```python
from build123d import *

# Parameters (mm, degrees)
SKETCH_W               = 9
SKETCH_H               = 250
PAD_DEPTH              = 6.5
SKETCH001_R            = 1.75
POCKET_DEPTH           = 6.5
LINEARPATTERN_COUNT    = 13
LINEARPATTERN_PITCH    = 20
SKETCH002_R            = 3
POCKET001_DEPTH        = 3.5
LINEARPATTERN001_COUNT = 13
LINEARPATTERN001_PITCH = 20
SKETCH005_W            = 20
SKETCH005_H            = 28.9
SKETCH005_R            = 1.75
PAD002_DEPTH           = 8


with BuildPart() as part:
    # Sketch → Pad (new body)
    with BuildSketch(Plane.XY):
        with Locations((0, 125)):
            Rectangle(SKETCH_W, SKETCH_H)
    extrude(amount=-PAD_DEPTH)

    # Sketch001 → Pocket (cut)
    with BuildSketch(Plane.XY):
        with Locations((0, 5)):
            Circle(SKETCH001_R)
    pocket = extrude(amount=-POCKET_DEPTH, mode=Mode.SUBTRACT)

    # LinearPattern: Pocket ×13
    with Locations(*[(0, i * LINEARPATTERN_PITCH, 0) for i in range(1, LINEARPATTERN_COUNT)]):
        add(pocket, mode=Mode.SUBTRACT)

    # Sketch002 → Pocket001 (cut)
    with BuildSketch(Plane.XY):
        with Locations((0, 5)):
            Circle(SKETCH002_R)
    pocket001 = extrude(amount=-POCKET001_DEPTH, mode=Mode.SUBTRACT)

    # LinearPattern001: Pocket001 ×13
    with Locations(*[(0, i * LINEARPATTERN001_PITCH, 0) for i in range(1, LINEARPATTERN001_COUNT)]):
        add(pocket001, mode=Mode.SUBTRACT)

    # Sketch005 → Pad002 (join)
    with BuildSketch(Plane.XY.offset(-4.5)):
        with Locations((0, 132.225)):
            Rectangle(SKETCH005_W, SKETCH005_H)
        with Locations((-7.5, 137.225)):
            Circle(SKETCH005_R, mode=Mode.SUBTRACT)
        with Locations((7.5, 137.225)):
            Circle(SKETCH005_R, mode=Mode.SUBTRACT)
        with Locations((7.5, 127.225)):
            Circle(SKETCH005_R, mode=Mode.SUBTRACT)
        with Locations((-7.5, 127.225)):
            Circle(SKETCH005_R, mode=Mode.SUBTRACT)
    extrude(amount=PAD002_DEPTH)


solid = part.part
```
Part model, mm, in its own coordinate system. A direction names the side the tool comes from. Coordinates: 2 decimals unless noted, no trailing zeros. Order: outer loops, then holes, each group sorted by start corner. A loop starts at its lowest first (then second) coordinate and runs counter-clockwise, first axis right, second up. Notation, with made-up numbers: (0.5, 57.25) - (20.5, 57.25) arc R20 ccw to (20.5, 65.25) - close; hole circle Ø8 at (16, 68.25). An arc over 180 degrees is marked (long way). Return JSON: item names as keys, results as strings. Group by question number.
Item 1: Pin check, flat tips, straight feed: pin 1 (3 mm diameter, centred on x = -1.5, y = 164, fed in from +Z); pin 2 (4 mm diameter, centred on x = 7.5, y = 84, fed in from +Z); pin 3 (1.7 mm diameter, centred on x = 0, y = 145, fed in from -Z); pin 4 (5.5 mm diameter, centred on x = 0, y = 205, fed in from +Z). Stop position of each tip, or through.
Item 2: Cut at A-A (z = 1.75). List the corners of the cut face in (x, y) (3 decimals), plus the area to 3 significant figures.
Item 3: Drill centre lines: probe 1 along Y at (x, z) = (-7.5, 1.75) (3 decimals); probe 2 along X at (y, z) = (185, -5.05); probe 3 along X at (y, z) = (137.5, -3). Where is each one in solid material? Low to high. Write a range as from..to.
Item 4: Which spindle directions (+Z, -Z, +X, -X, +Y, -Y) get a long thin tool onto all of the face, cutting with end or side? Do faces 4 (the face through (2, 245, -3.5)), 5 (the face through (0, 127, -6.5)), 6 (the face through (0, 199, 0)). Say none if no direction does.
Item 5: Pull direction Y, two halves, no side cores. Call faces 1 (the face through (10, 132, -1)), 2 (the face through (0, 250, -3)), 3 (the face through (2, 5, -3.5)): pulls with the +Y half, pulls with the -Y half, needs draft (parallel to the pull), parting line crosses it, or undercut.
Item 6: Cut at B-B (y = 175). List the corners of the cut face in (x, z), plus the area to 3 significant figures.
Check values:
{
 "1": {"pin 1": "stops at z = 0", "pin 2": "passes through", "pin 3": "stops at z = -4.5", "pin 4": "stops at z = -3.5"},
 "2": {"outline": "(-10, 117.775) - (10, 117.775) - (10, 146.675) - (-10, 146.675) - close; hole circle Ø3.5 at (-7.5, 127.225); hole circle Ø3.5 at (-7.5, 137.225); hole circle Ø3.5 at (7.5, 127.225); hole circle Ø3.5 at (7.5, 137.225)", "area": "540 mm2"},
 "3": {"probe 1": "y = 117.775..125.475, 128.975..135.475, 138.975..146.675", "probe 2": "x = -4.5..-1.75, 1.75..4.5", "probe 3": "x = -10..-9.23, -5.77..5.77, 9.23..10"},
 "4": {"face 4": "+Z", "face 5": "-Z, +X, -X, +Y, -Y", "face 6": "+Z, +X, -X, +Y"},
 "5": {"face 1": "needs draft", "face 2": "pulls with the +Y half", "face 3": "undercut"},
 "6": {"outline": "(-4.5, -6.5) - (4.5, -6.5) - (4.5, 0) - (-4.5, 0) - close", "area": "58.5 mm2"}
}
